from build123d import *

# Parameters (mm, degrees)
F1_DEPTH = 14.224
F2_DEPTH = 7.874
F3_DEPTH = 14.224
F0_W     = 6.35
F0_H     = 28.448
F4_DEPTH = 7.874


with BuildPart() as f1:
    # F0 (on Front) → F1 (new body, symmetric)
    with BuildSketch(Plane.XZ):
        Polygon((-4.571382422, -16.002), (-4.571382422, 16.002), (-70.6115919133, 16.002), (-76.9615919133, 16.002), (-76.9615919133, -16.002), (-70.6115919133, -16.002), align=None)
    extrude(amount=F1_DEPTH, both=True)

    # F0 (on Front) → F2 (join, symmetric)
    with BuildSketch(Plane.XZ):
        Polygon((-4.571382422, 16.002), (-0.7615919133, 16.002), (10.1604080867, 26.924), (-6.7215473391, 26.924), (-6.7215473391, 44.45), (-70.6115919133, 44.45), (-70.6115919133, 16.002), align=None)
        with BuildLine():
            ThreePointArc((-22.8595919133, 35.814), (-17.2715919133, 30.226), (-22.8595919133, 24.638))
            Line((-22.8595919133, 24.638), (-46.7355919133, 24.638))
            ThreePointArc((-46.7355919133, 24.638), (-52.3235919133, 30.226), (-46.7355919133, 35.814))
            Line((-46.7355919133, 35.814), (-22.8595919133, 35.814))
        make_face(mode=Mode.SUBTRACT)
        Polygon((-0.7615919133, -16.002), (-4.571382422, -16.002), (-70.6115919133, -16.002), (-70.6115919133, -44.45), (-6.7215473391, -44.45), (-6.7215473391, -26.924), (10.1604080867, -26.924), align=None)
        with BuildLine():
            Line((-22.8595919133, -35.814), (-46.7355919133, -35.814))
            ThreePointArc((-46.7355919133, -35.814), (-52.3235919133, -30.226), (-46.7355919133, -24.638))
            Line((-46.7355919133, -24.638), (-22.8595919133, -24.638))
            ThreePointArc((-22.8595919133, -24.638), (-17.2715919133, -30.226), (-22.8595919133, -35.814))
        make_face(mode=Mode.SUBTRACT)
    extrude(amount=F2_DEPTH, both=True)

    # F0 (on Front) → F3 (join, symmetric)
    with BuildSketch(Plane.XZ):
        Polygon((27.6864080867, -44.45), (10.1604080867, -26.924), (-6.7215473391, -26.924), (-6.7215473391, -44.45), align=None)
        Polygon((-6.7215473391, 26.924), (10.1604080867, 26.924), (27.6864080867, 44.45), (-6.7215473391, 44.45), align=None)
    extrude(amount=F3_DEPTH, both=True)

    # F0 (on Front) → F4 (join)
    with BuildSketch(Plane.XZ):
        with Locations((-73.7865919133, 30.226)):
            Rectangle(F0_W, F0_H)
        with Locations((-73.7865919133, -30.226)):
            Rectangle(F0_W, F0_H)
    extrude(amount=-F4_DEPTH)


solid = f1.part
Work out the finished part from the listing and answer in its coordinate system (mm). A direction names the side the tool comes from. Coordinates: 2 decimals unless noted, no trailing zeros. Write each loop counter-clockwise with the first axis right and the second up, starting at its lowest first coordinate (ties: lowest second). Pieces come first, ordered by that corner, then holes.
1. The part is cut by section A-A, the plane y = -10. Write down the section's boundary in (x, z).
Results list:
outline: (-76.96, -16) - (-4.57, -16) - (-4.57, 16) - (-76.96, 16) - close; (-6.72, -44.45) - (27.69, -44.45) - (10.16, -26.92) - (-6.72, -26.92) - close; (-6.72, 26.92) - (10.16, 26.92) - (27.69, 44.45) - (-6.72, 44.45) - close
2. Consider line 1 along Z through (x, y) = (-23.5, -4.25); line 2 along Z through (x, y) = (-3, -0.25); line 3 along X through (y, z) = (-6.25, 5.5). Determine where each line is inside the solid, lowest interval first.
Results list:
line 1: z = -44.45 to -35.81, -24.64 to 24.64, 35.81 to 44.45
line 2: z = -44.45 to -16, 16 to 44.45
line 3: x = -76.96 to -4.57
3. Flat-ended cylindrical pins translate along their axes: pin 1 (8 mm diameter, centred on y = -8.5, z = -22, fed in from +X); pin 2 (1.9 mm diameter, centred on y = -10.5, z = -34.5, fed in from -X); pin 3 (8 mm diameter, centred on y = 7.5, z = -6.5, fed in from +X). Find the tip coordinate at first contact, or state that the pin passes through.
Results list:
pin 1: stops at x = 9.19
pin 2: stops at x = -6.72
pin 3: stops at x = -4.57
4. The part is cut by section B-B, the plane x = -30. Write down the section's boundary in (y, z).
Results list:
outline: (-14.22, -16) - (-7.87, -16) - (-7.87, -24.64) - (7.87, -24.64) - (7.87, -16) - (14.22, -16) - (14.22, 16) - (7.87, 16) - (7.87, 24.64) - (-7.87, 24.64) - (-7.87, 16) - (-14.22, 16) - close; (-7.87, -44.45) - (7.87, -44.45) - (7.87, -35.81) - (-7.87, -35.81) - close; (-7.87, 35.81) - (7.87, 35.81) - (7.87, 44.45) - (-7.87, 44.45) - close
5. For a pull along Z with two mould halves and no side action, classify faces 4 (the flat face through (-76.962, 0, -1)), 5 (the flat face through (2, 11, -26.924)), 6 (the flat face through (-3, 0, -16.002)), 7 (the flat face through (-14, 0, -44.45)) as +Z half, -Z half, draft (parallel to the pull), parting line (faces both ways), or undercut.
Results list:
face 4: draft
face 5: undercut
face 6: undercut
face 7: -Z half
6. The part is cut by section C-C, the plane y = 2.25. Write down the section's boundary in (x, z), and give its area (3 significant figures).
Results list:
outline: (-76.96, -44.45) - (27.69, -44.45) - (-0.76, -16) - (-4.57, -16) - (-4.57, 16) - (-0.76, 16) - (27.69, 44.45) - (-76.96, 44.45) - close; hole (-46.74, -35.81) - (-22.86, -35.81) arc R5.59 ccw to (-22.86, -24.64) - (-46.74, -24.64) arc R5.59 ccw to start; hole (-46.74, 24.64) - (-22.86, 24.64) arc R5.59 ccw to (-22.86, 35.81) - (-46.74, 35.81) arc R5.59 ccw to start
area: 6,730 mm2
7. For faces 1 (the flat face through (-6.722, 11, -36)), 2 (the flat face through (2, 11, 26.924)), 3 (the flat face through (-74, 0, 30)), determine the directions among +Z, -Z, +X, -X, +Y, -Y from which every point of the face is accessible in a straight line to the end or side of a thin tool.
Results list:
face 1: -Z, -X, +Y
face 2: +X, -X, +Y
face 3: +Z, -X, -Y
8. The part is cut by section D-D, the plane x = -61. Write down the section's boundary in (y, z).
Results list:
outline: (-14.22, -16) - (-7.87, -16) - (-7.87, -44.45) - (7.87, -44.45) - (7.87, -16) - (14.22, -16) - (14.22, 16) - (7.87, 16) - (7.87, 44.45) - (-7.87, 44.45) - (-7.87, 16) - (-14.22, 16) - close
